```python
from build123d import *

# Parameters (mm, degrees)
PAD_DEPTH       = 25
SKETCH001_W     = 25
SKETCH001_H     = 40
POCKET_DEPTH    = 63.001
POCKET001_DEPTH = 429.133955
FILLET_R        = 10
SKETCH003_R     = 4
POCKET002_DEPTH = 53.001


with BuildPart() as part:
    # Sketch → Pad (new body, symmetric)
    with BuildSketch(Plane.YZ):
        Polygon((-107, 0), (0, 0), (0, -45), (8, -45), (8, 0), (63, 0), (63, 8), (23, 8), (13, 18), (-77, 18), (-82, 13), (-82, 8), (-102, 8), (-107, 2), align=None)
    extrude(amount=PAD_DEPTH, both=True)

    # Sketch001 → Pocket (cut, through all)
    with BuildSketch(Plane(origin=(0, 0, 0), x_dir=(0, 0, -1), z_dir=(0, -1, 0))):
        with Locations((27.5, 0)):
            Rectangle(SKETCH001_W, SKETCH001_H)
    extrude(amount=-POCKET_DEPTH, mode=Mode.SUBTRACT)

    # Sketch002 → Pocket001 (cut, through all)
    with BuildSketch(Plane(origin=(0, 0, 8), x_dir=(0, -1, 0), z_dir=(0, 0, 1))):
        Polygon((-22.911764, -25), (-63, 0), (-63, -25), align=None)
    pocket001 = extrude(amount=-POCKET001_DEPTH, mode=Mode.SUBTRACT)

    # Mirrored: Pocket001 across Sketch002 H_Axis
    add(pocket001.mirror(Plane(origin=(0, 0, 8), x_dir=(0, 0, 1), z_dir=(1, 0, 0))), mode=Mode.SUBTRACT)

    # Fillet
    fillet_edges = [part.edges().sort_by_distance(p)[0] for p in [
        (0, 63, 4),
    ]]
    fillet(fillet_edges, radius=FILLET_R)

    # Sketch003 → Pocket002 (cut, through all)
    with BuildSketch(Plane(origin=(0, 0, 8), x_dir=(0, -1, 0), z_dir=(0, 0, 1))):
        with Locations((-44.102099, 0)):
            Circle(SKETCH003_R)
    extrude(amount=-POCKET002_DEPTH, mode=Mode.SUBTRACT)


solid = part.part
```
Source: CAD feature listing. Evaluate the final solid. Frame: model axes, mm. A direction names the side the tool comes from. Coordinates: 2 decimals unless noted, no trailing zeros. Loops run counter-clockwise (first coordinate to the right, second up) from the corner with the lowest first, then second, coordinate; pieces in that order, holes last. Notation, with made-up numbers: M 61.5,-28.75 L 90.5,-28.75 A18 ccw 90.5,-10.75 Z; hole C 78.5,27.5 d4. An arc over 180 degrees is marked long. Use a Markdown table: item, result. Add a question column.
Q1. Section query B-B, the plane x = 0. Return loops of the section in (y, z), and give its area (3 significant figures).
Q2. Section query C-C, the plane x = 14. Return loops of the section in (y, z), and give its area (3 significant figures).
Q3. Access query for faces 1 (the flat face through (0, 8, -13)), 2 (the flat face through (0, 4, -15)), 3 (the flat face through (0, -92, 8)). Directions: +Z, -Z, +X, -X, +Y, -Y. A direction counts if a zero-diameter tool reaches every point of the face in a straight line with its end or side. Return the directions, or none.
Q4. First-contact query: pin 1 (1.5 mm diameter, centred on x = 0, z = 11, fed in from -Y); pin 2 (3 mm diameter, centred on x = -0.5, y = -88.5, fed in from +Z); pin 3 (1 mm diameter, centred on x = -4, z = -9.5, fed in from +Y). Flat tips, straight axial feed; report the tip coordinate or a pass-through.
Q5. Section query A-A, the plane z = -36.5. Return loops of the section in (x, y), and give its area (3 significant figures).
Q6. Section query D-D, the plane z = -4. Return loops of the section in (x, y).
Q7. Draft query along Z for faces 4 (the flat face through (0, 35, 8)), 5 (the flat face through (0, -82, 11)), 6 (the flat face through (20, 4, -27)). Return one class per face: pulls with the +Z half, pulls with the -Z half, needs draft (parallel to the pull), parting line crosses it, or undercut.
Q8. Material intervals for L1, parallel to X at y = 1, z = -27; L2, parallel to Z at x = 6, y = -97.5, sorted ascending.
Result:
| question | item | result |
|---|---|---|
| 1 | outline | M -107,0 L 0,0 L 0,-15 L 8,-15 L 8,0 L 40.1,0 L 40.1,8 L 23,8 L 13,18 L -77,18 L -82,13 L -82,8 L -102,8 L -107,2 Z; M 0,-45 L 8,-45 L 8,-40 L 0,-40 Z; M 48.1,0 L 54.1,0 L 54.1,8 L 48.1,8 Z |
| 1 | area | 2,360 mm2 |
| 2 | outline | M -107,0 L 0,0 L 0,-15 L 8,-15 L 8,0 L 40.55,0 L 40.55,8 L 23,8 L 13,18 L -77,18 L -82,13 L -82,8 L -102,8 L -107,2 Z; M 0,-45 L 8,-45 L 8,-40 L 0,-40 Z |
| 2 | area | 2,310 mm2 |
| 3 | face 1 | -Z, +X, -X, +Y |
| 3 | face 2 | +Y, -Y |
| 3 | face 3 | +Z, +X, -X, -Y |
| 4 | pin 1 | stops at y = -82 |
| 4 | pin 2 | stops at z = 8 |
| 4 | pin 3 | stops at y = 8 |
| 5 | outline | M -25,0 L -20,0 L -20,8 L -25,8 Z; M 20,0 L 25,0 L 25,8 L 20,8 Z |
| 5 | area | 80.0 mm2 |
| 6 | outline | M -25,0 L 25,0 L 25,8 L -25,8 Z |
| 7 | face 4 | pulls with the +Z half |
| 7 | face 5 | needs draft |
| 7 | face 6 | undercut |
| 8 | L1 | x = -25 to -20, 20 to 25 |
| 8 | L2 | z = 0 to 8 |
